Work out the finished part from the listing and answer in its coordinate system (mm). A direction names the side the tool comes from. Round coordinates to 2 decimals unless told otherwise and drop trailing zeros. Write each loop counter-clockwise with the first axis right and the second up, starting at its lowest first coordinate (ties: lowest second). Pieces come first, ordered by that corner, then holes. Notation, with made-up numbers: M 34.25,-33 L 69.25,-33 A18 ccw 69.25,0 Z; hole C 8,-31 d9. An arc over 180 degrees is marked long. Answer in a Markdown table with one row per item.
```python
from build123d import *

# Parameters (mm, degrees)
CORTAR_EXTRUIR1_DEPTH      = 88.241045386
CORTAR_EXTRUIR1_DEPTH_BACK = 88.241045386
CROQUIS2_R                 = 3
CORTAR_EXTRUIR2_DEPTH      = 88.241045559
CORTAR_EXTRUIR2_DEPTH_BACK = 88.241045559
CROQUIS3_R                 = 3
CORTAR_EXTRUIR3_DEPTH      = 88.241045559
CORTAR_EXTRUIR3_DEPTH_BACK = 88.241045559
CROQUIS4_R                 = 3
CORTAR_EXTRUIR4_DEPTH      = 88.241045559
CORTAR_EXTRUIR4_DEPTH_BACK = 88.241045559
CROQUIS5_R                 = 3


with BuildPart() as part:
    # Croquis1 → Revolución1 (revolve)
    with BuildSketch(Plane(origin=(0, 0, 0), x_dir=(0, 0, -1), z_dir=(1, 0, 0)), mode=Mode.PRIVATE) as revoluci_n1_sk:
        Polygon((-49, 53), (-36, 53), (-36, 34), (-39, 34), (-39, 14), (-49, 14), align=None)
    revolve(revoluci_n1_sk.sketch.rotate(Axis((0, 0, 0), (0, 1, 0)), 180), axis=Axis((0, 0, 0), (0, 1, 0)))

    # Croquis2 → Cortar-Extruir1 (cut, two sides: drawn at the far end of the back side and taken through both)
    with BuildSketch(Plane(origin=(0, 0, 0), x_dir=(0, 0, -1), z_dir=(1, 0, 0)).offset(-CORTAR_EXTRUIR1_DEPTH_BACK)):
        with Locations((0, 38)):
            Circle(CROQUIS2_R)
    extrude(amount=CORTAR_EXTRUIR1_DEPTH + CORTAR_EXTRUIR1_DEPTH_BACK, mode=Mode.SUBTRACT)

    # Croquis3 → Cortar-Extruir2 (cut, two sides: drawn at the far end of the back side and taken through both)
    with BuildSketch(Plane.XY.offset(-CORTAR_EXTRUIR2_DEPTH_BACK)):
        with Locations((0, 38)):
            Circle(CROQUIS3_R)
    extrude(amount=CORTAR_EXTRUIR2_DEPTH + CORTAR_EXTRUIR2_DEPTH_BACK, mode=Mode.SUBTRACT)

    # Croquis4 → Cortar-Extruir3 (cut, two sides: drawn at the far end of the back side and taken through both)
    with BuildSketch(Plane(origin=(0, 0, 0), x_dir=(-0.7071067811865477, 0, -0.7071067811865475), z_dir=(0.7071067811865475, 0, -0.7071067811865477)).offset(-CORTAR_EXTRUIR3_DEPTH_BACK)):
        with Locations((0, 38.362139971)):
            Circle(CROQUIS4_R)
    extrude(amount=CORTAR_EXTRUIR3_DEPTH + CORTAR_EXTRUIR3_DEPTH_BACK, mode=Mode.SUBTRACT)

    # Croquis5 → Cortar-Extruir4 (cut, two sides: drawn at the far end of the back side and taken through both)
    with BuildSketch(Plane(origin=(0, 0, 0), x_dir=(0.7071067811865502, 0, -0.7071067811865449), z_dir=(0.7071067811865449, 6.982962677686268e-15, 0.7071067811865502)).offset(-CORTAR_EXTRUIR4_DEPTH_BACK)):
        with Locations((0, 38)):
            Circle(CROQUIS5_R)
    extrude(amount=CORTAR_EXTRUIR4_DEPTH + CORTAR_EXTRUIR4_DEPTH_BACK, mode=Mode.SUBTRACT)


solid = part.part
```
1. The part is cut by section D-D (x = -11.5). Determine the outline of the cut face in (y, z).
Calculated:
| item | result |
|---|---|
| outline | M 14,-47.63 L 53,-47.63 L 53,-34.11 L 34,-34.11 L 34,-37.27 L 14,-37.27 Z; M 14,37.27 L 34,37.27 L 34,34.11 L 53,34.11 L 53,47.63 L 14,47.63 Z |
2. Determine the mould class of faces 3 (the cylindrical face through (-38.668, 23.86, 5.077)), 4 (the flat face through (22, 14, -33)), 5 (the cylindrical face through (42, 41, 0)) for opening direction Y: released by +Y, released by -Y, zero draft, split by the parting line, or undercut.
Calculated:
| item | result |
|---|---|
| face 3 | zero draft |
| face 4 | released by -Y |
| face 5 | undercut |
3. Given pin 1 (1.5 mm diameter, centred on y = 44, z = 28, fed in from -X); pin 2 (3 mm diameter, centred on x = -4.5, y = 20, fed in from +Z); pin 3 (10 mm diameter, centred on y = 48, z = -5.5, fed in from +X), each flat-ended and moving along its own axis, determine where each tip first touches the part or whether it passes through.
Calculated:
| item | result |
|---|---|
| pin 1 | stops at x = -40.72 |
| pin 2 | stops at z = 48.91 |
| pin 3 | stops at x = 49 |
4. The part is cut by section B-B (x = 0). Determine the outline of the cut face in (y, z).
Calculated:
| item | result |
|---|---|
| outline | M 14,-49 L 35,-49 L 35,-36 L 34,-36 L 34,-39 L 14,-39 Z; M 14,39 L 34,39 L 34,36 L 35,36 L 35,49 L 14,49 Z; M 41,-49 L 53,-49 L 53,-36 L 41,-36 Z; M 41,36 L 53,36 L 53,49 L 41,49 Z |
5. A tool of negligible diameter and unlimited length cuts with its end or side. For faces 1 (the flat face through (34.5, 34, 11.4)), 2 (the cylindrical face through (18.767, 33.773, -45.264)), from which of +Z, -Z, +X, -X, +Y, -Y can it reach the whole face along a straight path? Write none if from no direction.
Calculated:
| item | result |
|---|---|
| face 1 | -Y |
| face 2 | +Y, -Y |
6. Consider line 1 along Y through (x, z) = (-39.25, 0); line 2 along Y through (x, z) = (26, 26); line 3 along X through (y, z) = (25, 0). Determine where each line is inside the solid, lowest interval first. Write a range as from..to.
Calculated:
| item | result |
|---|---|
| line 1 | y = 14..35, 41..53 |
| line 2 | y = 34..35, 41..53 |
| line 3 | x = -49..-39, 39..49 |
7. The part is cut by section C-C (y = 48.5). Determine the outline of the cut face in (x, z).
Calculated:
| item | result |
|---|---|
| outline | C 0,0 d98; hole C 0,0 d72 |
8. The part is cut by section A-A (z = 0). Determine the outline of the cut face in (x, y).
Calculated:
| item | result |
|---|---|
| outline | M -49,14 L -39,14 L -39,34 L -36,34 L -36,35 L -49,35 Z; M -49,41 L -36,41 L -36,53 L -49,53 Z; M 36,34 L 39,34 L 39,14 L 49,14 L 49,35 L 36,35 Z; M 36,41 L 49,41 L 49,53 L 36,53 Z |
